from build123d import *

# Parameters (mm, degrees)
SKETCH1_W           = 20.3
SKETCH1_H           = 20.3
SKETCH1_W_2         = 16.3
SKETCH1_H_2         = 16.3
BOSS_EXTRUDE1_DEPTH = 25
SKETCH2_W           = 20.3
SKETCH2_H           = 20.3
SKETCH2_W_2         = 14
SKETCH2_H_2         = 14
BOSS_EXTRUDE2_DEPTH = 3
SKETCH3_R           = 1
SKETCH3_R_2         = 2.5
CUT_EXTRUDE1_DEPTH  = 34.765551972
FILLET1_R           = 1


with BuildPart() as part:
    # Sketch1 → Boss-Extrude1 (new body)
    with BuildSketch(Plane.XY):
        Rectangle(SKETCH1_W, SKETCH1_H)
        Rectangle(SKETCH1_W_2, SKETCH1_H_2, mode=Mode.SUBTRACT)
    extrude(amount=-BOSS_EXTRUDE1_DEPTH)

    # Sketch2 → Boss-Extrude2 (add)
    with BuildSketch(Plane.XY):
        Rectangle(SKETCH2_W, SKETCH2_H)
        Rectangle(SKETCH2_W_2, SKETCH2_H_2, mode=Mode.SUBTRACT)
    extrude(amount=BOSS_EXTRUDE2_DEPTH)

    # Sketch3 → Cut-Extrude1 (cut, through all)
    with BuildSketch(Plane(origin=(10.15, 0, 0), x_dir=(0, 0, -1), z_dir=(1, 0, 0))):
        with Locations((20.5, 0)):
            Circle(SKETCH3_R)
        with Locations((9.5, 0)):
            Circle(SKETCH3_R_2)
    extrude(amount=-CUT_EXTRUDE1_DEPTH, mode=Mode.SUBTRACT)

    # Fillet1
    fillet1_edges = [part.edges().sort_by_distance(p)[0] for p in [
        (8.15, 0, -25),
        (0, -8.15, -25),
        (-8.15, 0, -25),
        (0, 8.15, -25),
    ]]
    fillet(fillet1_edges, radius=FILLET1_R)


solid = part.part
Can you work these out from the model? Positions are in its coordinate system, mm. A direction names the side the tool comes from. Coordinates: 2 decimals unless noted, no trailing zeros. Loops run counter-clockwise (first coordinate to the right, second up) from the corner with the lowest first, then second, coordinate; pieces in that order, holes last. Notation, with made-up numbers: M 74,5.5 L 120,5.5 A19 ccw 120,29.5 Z; hole C 16.25,58.5 d5. An arc over 180 degrees is marked long. Return JSON: item names as keys, results as strings. Group by question number.
Item 1: On a 3-axis mill with a long thin cutter (end or side, diameter ignored), from which of +Z, -Z, +X, -X, +Y, -Y can I reach the whole of each face in a straight line? I mean faces 4 (the cylindrical face through (-8.451, 0.128, -24.715)), 5 (the flat face through (0, 7, 1)), 6 (the flat face through (10.15, -2.4, -11.2)). Say none if no direction works.
Item 2: Thinking about a two-plate mould opening in X: for faces 1 (the flat face through (-10.15, -2.4, -11.2)), 2 (the flat face through (0, -8.15, -12)), 3 (the cylindrical face through (9, 0, -7)), which applies, released by +X, released by -X, zero draft, split by the parting line, or undercut?
Item 3: Imagine slicing it at C-C (z = -9.5). Please give me the cut outline in (x, y).
Item 4: Imagine slicing it at A-A (y = -4.5). Please give me the cut outline in (x, z), and give its area (3 significant figures).
Item 5: If I drill on L1, parallel to Y at x = -4.25, z = -3.25; L2, parallel to Y at x = -8.7, z = -9.5, over which ranges is the centre line in solid material (lowest first)? Write a range as from..to.
Item 6: I'm going to push a flat-ended pin straight in: pin 1 Ø1.6 at (y, z) = (0, -20.5) entering from +X. Where does the tip first touch, or does it pass through?
Item 7: Imagine slicing it at D-D (y = 0). Give the number of separate pieces and of enclosed holes in the cut face, and give its area (3 significant figures).
Verdict:
{
 "1": {"face 4": "-Z", "face 5": "+Z, -Z", "face 6": "+Z, -Z, +X, +Y, -Y"},
 "2": {"face 1": "released by -X", "face 2": "undercut", "face 3": "zero draft"},
 "3": {"outline": "M -10.15,-10.15 L 10.15,-10.15 L 10.15,-2.5 L 8.15,-2.5 L 8.15,-8.15 L -8.15,-8.15 L -8.15,-2.5 L -10.15,-2.5 Z; M -10.15,2.5 L -8.15,2.5 L -8.15,8.15 L 8.15,8.15 L 8.15,2.5 L 10.15,2.5 L 10.15,10.15 L -10.15,10.15 Z"},
 "4": {"outline": "M -10.15,-25 L -9.15,-25 A1 ccw -8.15,-24 L -8.15,0 L -7,0 L -7,3 L -10.15,3 Z; M 7,0 L 8.15,0 L 8.15,-24 A1 ccw 9.15,-25 L 10.15,-25 L 10.15,3 L 7,3 Z", "area": "118 mm^2"},
 "5": {"L1": "y = -10.15..-8.15, 8.15..10.15", "L2": "y = -10.15..-2.5, 2.5..10.15"},
 "6": {"pin 1": "passes through"},
 "7": {"separate pieces": "6", "enclosed holes": "0", "area": "90.5 mm^2"}
}
